Answer from the drawing. Dimensions are ordinates in mm from the lowest x, y and z of the part. A direction names the side the tool comes from. Coordinates: 2 decimals unless noted, no trailing zeros. Write each loop counter-clockwise with the first axis right and the second up, starting at its lowest first coordinate (ties: lowest second). Pieces come first, ordered by that corner, then holes. Notation, with made-up numbers: (82, 41.5) -> (139, 41.5) arc R34 ccw to (139, 78.5) -> close; hole circle Ø5 at (43, 14.5). An arc over 180 degrees is marked (long way). Answer as a JSON object with one key per item and string values. Group by question number.
(1) Find section C-C (y = 20.5). Give the vertices of the cut face in (x, z), then the cut area to 3 significant figures.
(2) Find section B-B (z = 23.75). Give the vertices of the cut face in (x, y), then the cut area to 3 significant figures.
(3) For a pull along X with two mould halves and no side action, classify the marked faces 1, 2 and 3 as +X half, -X half, draft (parallel to the pull), parting line (faces both ways), or undercut.
(4) Which of the six approach directions +Z, -Z, +X, -X, +Y, -Y give full straight-line access (tool end or side, diameter ignored) to the marked faces 4 and 5?
(5) Straight lines are drawn through the part: L1, parallel to Z at x = 54, y = 22.5; L2, parallel to X at y = 23, z = 24.5; L3, parallel to Y at x = 47, z = 27. For each, find the intervals that lie inside material, in ascending order.
(6) Find section D-D (x = 40.35). Give the vertices of the cut face in (y, z), then the cut area to 3 significant figures.
(7) Flat-ended cylindrical pins translate along their axes: P1, Ø10, axis at x = 52.5, y = 19, coming from the +Z side; P2, Ø5, axis at y = 31, z = 24, coming from the +X side; P3, Ø1.5, axis at y = 29.5, z = 24, coming from the +X side. Find the tip coordinate at first contact, or state that the pin passes through.
(8) Find section A-A (x = 13.12). Give the vertices of the cut face in (y, z), then the cut area to 3 significant figures.
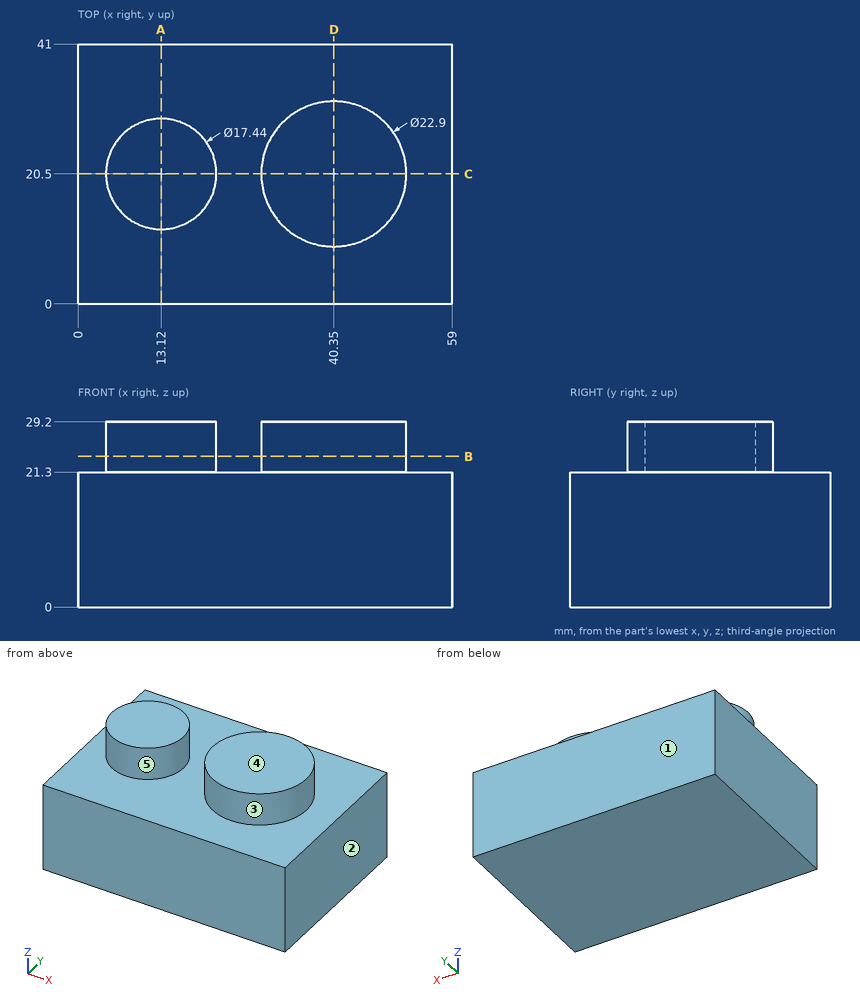
Results below:
{
 "1": {"outline": "(0, 0) -> (59, 0) -> (59, 21.3) -> (51.8, 21.3) -> (51.8, 29.2) -> (28.9, 29.2) -> (28.9, 21.3) -> (21.84, 21.3) -> (21.84, 29.2) -> (4.4, 29.2) -> (4.4, 21.3) -> (0, 21.3) -> close", "area": "1,580 mm2"},
 "2": {"outline": "circle Ø17.44 at (13.12, 20.5); circle Ø22.9 at (40.35, 20.5)", "area": "651 mm2"},
 "3": {"face 1": "draft", "face 2": "+X half", "face 3": "undercut"},
 "4": {"face 4": "+Z, +X, -X, +Y, -Y", "face 5": "+Z"},
 "5": {"L1": "z = 0 to 21.3", "L2": "x = 4.77 to 21.47, 29.18 to 51.52", "L3": "y = 11.18 to 29.82"},
 "6": {"outline": "(0, 0) -> (41, 0) -> (41, 21.3) -> (31.95, 21.3) -> (31.95, 29.2) -> (9.05, 29.2) -> (9.05, 21.3) -> (0, 21.3) -> close", "area": "1,050 mm2"},
 "7": {"P1": "stops at z = 29.2", "P2": "stops at x = 48.54", "P3": "stops at x = 48.29"},
 "8": {"outline": "(0, 0) -> (41, 0) -> (41, 21.3) -> (29.22, 21.3) -> (29.22, 29.2) -> (11.78, 29.2) -> (11.78, 21.3) -> (0, 21.3) -> close", "area": "1,010 mm2"}
}
